Build history of the part. All positions in model axes, mm. A direction names the side the tool comes from. Give positions to 0.01 mm unless a question says otherwise; leave off trailing zeros. Loops run counter-clockwise (first coordinate to the right, second up) from the corner with the lowest first, then second, coordinate; pieces in that order, holes last. Notation, with made-up numbers: M 50,56 L 98,56 A14 ccw 98,76 Z; hole C -24.5,-3.75 d6. An arc over 180 degrees is marked long. Put each result on its own line as item: value.
```python
from build123d import *

# Parameters (mm, degrees)
BOSS_EXTRUDE1_DEPTH = 20
BOSS_EXTRUDE2_DEPTH = 3
BOSS_EXTRUDE3_DEPTH = 3
SKETCH4_R           = 2.1
CUT_EXTRUDE1_DEPTH  = 63.040309477
SKETCH5_R           = 2
CUT_EXTRUDE2_DEPTH  = 3
FILLET3_R           = 2
FILLET4_R           = 0.5


with BuildPart() as part:
    # Sketch1 → Boss-Extrude1 (new body)
    with BuildSketch(Plane.XY):
        Polygon((0, 0), (0, 43), (3, 43), (3, 3), (43, 3), (43, 0), align=None)
    extrude(amount=BOSS_EXTRUDE1_DEPTH)

    # Sketch2 → Boss-Extrude2 (add)
    with BuildSketch(Plane.XY.offset(20)):
        Polygon((3, 43), (43, 3), (3, 3), align=None)
    extrude(amount=-BOSS_EXTRUDE2_DEPTH)

    # Sketch3 → Boss-Extrude3 (add)
    with BuildSketch(Plane(origin=(0, 0, 0), x_dir=(-1, 0, 0), z_dir=(0, 0, -1))):
        Polygon((-3, 43), (-43, 3), (-3, 3), align=None)
    extrude(amount=-BOSS_EXTRUDE3_DEPTH)

    # Sketch4 → Cut-Extrude1 (cut, through all)
    with BuildSketch(Plane(origin=(3, 0, 0), x_dir=(0, 0, -1), z_dir=(1, 0, 0))):
        with Locations(Location((-10, 33, 0), (0, 0, 90))):
            Circle(SKETCH4_R)
        with Locations(Location((-10, 13, 0), (0, 0, 90))):
            Circle(SKETCH4_R)
    extrude(amount=-CUT_EXTRUDE1_DEPTH, mode=Mode.SUBTRACT)

    # Sketch5 → Cut-Extrude2 (cut)
    with BuildSketch(Plane(origin=(0, 3, 0), x_dir=(1, 0, 0), z_dir=(0, 1, 0))):
        with Locations(Location((13, -10, 0), (0, 0, 270))):
            Circle(SKETCH5_R)
        with Locations(Location((33, -10, 0), (0, 0, 270))):
            Circle(SKETCH5_R)
    extrude(amount=-CUT_EXTRUDE2_DEPTH, mode=Mode.SUBTRACT)

    # Fillet3
    fillet3_edges = [part.edges().sort_by_distance(p)[0] for p in [
        (3, 3, 10),
        (3, 23, 17),
        (23, 3, 17),
        (3, 23, 3),
        (23, 3, 3),
    ]]
    fillet(fillet3_edges, radius=FILLET3_R)

    # Fillet4
    fillet4_edges = [part.edges().sort_by_distance(p)[0] for p in [
        (3, 30.9, 10),
        (3, 10.9, 10),
        (13, 3, 8),
        (33, 3, 8),
    ]]
    fillet(fillet4_edges, radius=FILLET4_R)


solid = part.part
```
Q1. Mould opens along Z. For faces 1 (the flat face through (17, 17, 20)), 2 (the cylindrical face through (3.6, 24.27, 3.57)), 3 (the flat face through (1, 43, 10)) say: pulls with the +Z half, pulls with the -Z half, needs draft (parallel to the pull), parting line crosses it, or undercut.
Here are the results:
face 1: pulls with the +Z half
face 2: undercut
face 3: needs draft
Q2. Slice it at D-D (y = 29). List the corners of the cut face in (x, z), and give its area (3 significant figures).
Here are the results:
outline: M 0,0 L 17,0 L 17,3 L 5,3 A2 cw 3,5 L 3,15 A2 cw 5,17 L 17,17 L 17,20 L 0,20 Z
area: 146 mm²
Q3. Tool access for faces 4 (the flat face through (23, 23, 1)), 5 (the flat face through (3, 24, 10)): list every direction of +Z, -Z, +X, -X, +Y, -Y with a clear straight run to the whole face (end or side of a thin tool).
Here are the results:
face 4: +Z, -Z, +X, +Y
face 5: +X, +Y
Q4. Slice it at B-B (x = 33). List the corners of the cut face in (y, z), and give its area (3 significant figures).
Here are the results:
outline: M 0,0 L 13,0 L 13,3 L 5,3 A2 cw 3,5 L 3,7.5 A0.5 ccw 2.5,8 L 0,8 Z; M 0,12 L 2.5,12 A0.5 ccw 3,12.5 L 3,15 A2 cw 5,17 L 13,17 L 13,20 L 0,20 Z
area: 110 mm²
Q5. Drop flat-ended pins along their axis: pin 1 Ø3 at (x, z) = (13, 10) entering from +Y; pin 2 Ø5 at (x, z) = (20.5, 9) entering from +Y; pin 3 Ø6 at (x, z) = (21, 7.5) entering from +Y; pin 4 Ø8 at (y, z) = (28, 11.5) entering from +X. Give the stop position or say it passes through.
Here are the results:
pin 1: through
pin 2: y = 3
pin 3: y = 3.06
pin 4: x = 3.06
Q6. Probe line 1 (X direction, y = 0.65, z = 10); line 2 (Z direction, x = 1.6, y = 33); line 3 (Z direction, x = 19.5, y = 22). List the from-to ranges inside material, lowest first. Write a range as from..to.
Here are the results:
line 1: 0..11, 15..31, 35..43
line 2: 0..7.9, 12.1..20
line 3: 0..3, 17..20
Q7. Slice it at A-A (z = 10). State how many separate pieces and enclosed holes the cut face has, and give its area (3 significant figures).
Here are the results:
separate pieces: 5
enclosed holes: 0
area: 200 mm²
Q8. Slice it at C-C (y = 13). List the corners of the cut face in (x, z).
Here are the results:
outline: M 0,0 L 33,0 L 33,3 L 5,3 A2 cw 3,5 L 3,7.4 A0.5 ccw 2.5,7.9 L 0,7.9 Z; M 0,12.1 L 2.5,12.1 A0.5 ccw 3,12.6 L 3,15 A2 cw 5,17 L 33,17 L 33,20 L 0,20 Z
